Verification items for the finished model (mm, model axes). A direction names the side the tool comes from. Give positions to 0.01 mm unless a question says otherwise; leave off trailing zeros. Loops run counter-clockwise (first coordinate to the right, second up) from the corner with the lowest first, then second, coordinate; pieces in that order, holes last. Notation, with made-up numbers: (18.5, 65.25) -> (46.5, 65.25) arc R9 cw to (46.5, 72.25) -> close; hole circle Ø6 at (4, -8.75). An arc over 180 degrees is marked (long way). Use one line per item in the form item = value. Start each with the question number.
from build123d import *

# Parameters (mm, degrees)
F0_W        = 7.45
F0_H        = 4
F1_DEPTH    = 2
F2_W        = 7.45
F2_H        = 5.9
F3_DEPTH    = 1.75
F6_W        = 7.45
F6_H        = 5
F7_DEPTH    = 2
F8_R        = 0.75
F9_T1_DEPTH = 1.05
F9_S5_W     = 0.75
F9_S5_H     = 0.75
F9_T6_DEPTH = 0.75


# Not quite as in the source:
# - a fillet or chamfer that OpenCascade refuses, or shapes differently, is made with other operations: its cross-section is extruded or revolved along the edge and cut away or added


with BuildPart() as f1:
    # F0 (on Top) → F1 (new body)
    with BuildSketch(Plane.XY):
        with Locations((3.725, 2)):
            Rectangle(F0_W, F0_H)
    extrude(amount=F1_DEPTH)

    # F2 (on face) → F3 (join)
    with BuildSketch(Plane.XY.offset(2)):
        with Locations((3.725, 2.85)):
            Rectangle(F2_W, F2_H)
    extrude(amount=F3_DEPTH)

    # F6 (on line) → F7 (join)
    with BuildSketch(Plane(origin=(0, 2.8829689891, 1.0493148984), x_dir=(-1, 0, 0), z_dir=(0, 0.9396926208, 0.3420201433))):
        with Locations((-3.725, 5.3740090556)):
            Rectangle(F6_W, F6_H)
    extrude(amount=-F7_DEPTH)

    # F8
    f8_edges = [f1.edges().sort_by_distance(p)[0] for p in [
        (7.45, 5.8, 2.875),
        (7.45, 3.85, 3.75),
        (3.725, 5.8, 3.75),
        (3.725, 5.8, 2),
        (0, 5.8, 2.875),
        (0, 3.85, 3.75),
        (0, 4.9, 2),
        (0, 1.04495, 6.099232),
        (3.725, 0.189899, 8.448463),
        (7.45, 1.04495, 6.099232),
        (7.45, -0.749793, 8.106443),
        (0, -0.749793, 8.106443),
    ]]
    fillet(f8_edges, radius=F8_R)

    # F9: fillet of radius 0.75 on 1 edges, made by hand

    # F9_s2 → F9_t1 (cut)
    with BuildSketch(Plane.XZ.offset(-5.05)):
        with BuildLine():
            ThreePointArc((7.45, 2.75), (7.2303300859, 2.2196699141), (6.7, 2))
            Line((6.7, 2), (7.45, 2))
            Line((7.45, 2), (7.45, 2.75))
        make_face()
    extrude(amount=F9_T1_DEPTH, mode=Mode.SUBTRACT)


with BuildPart() as f9_tool4:
    # F9_s5 → F9_t6 (new body)
    with BuildSketch(Plane.YZ.offset(6.7)):
        with Locations((5.425, 2.375)):
            Rectangle(F9_S5_W, F9_S5_H)
    extrude(amount=F9_T6_DEPTH)

    # F9_s7 → F9_t8 (revolve, cut)
    with BuildSketch(Plane(origin=(6.7, 5.05, 2.75), x_dir=(0, -0.7071067812, 0.7071067812), z_dir=(0, 0.7071067812, 0.7071067812))):
        with BuildLine():
            ThreePointArc((0, -0.75), (0.75, 0), (0, 0.75))
            Line((0, 0.75), (0, -0.75))
        make_face()
    revolve(axis=Axis((6.7, 5.05, 2.75), (1, 0, 0)), mode=Mode.SUBTRACT)


with BuildPart() as f1_1:
    add(f1.part)

    # F9_t3: cut F9_tool4
    add(f9_tool4.part, mode=Mode.SUBTRACT)


solid = f1_1.part
Item 1: Gauge pin test, flat ends, axial feed: pin 1 Ø0.8 at (x, z) = (5, 1) entering from +Y; pin 2 Ø1.5 at (x, z) = (2, 3) entering from -Y; pin 3 Ø2 at (x, y) = (6.5, 4) entering from +Z; pin 4 Ø1.2 at (x, y) = (4, 4.5) entering from -Z. Record the tip position at first contact, or that the pin passes through.
Item 2: Tool access check on faces 1 (the flat face through (4, -0.1, 3)), 2 (the flat face through (3.7, 4.5, 2)), 3 (the cylindrical face through (0.21, 1.04, 5.45)), 4 (the flat face through (4, 3, 3.75)), 5 (the cylindrical face through (3.68, 0.07, 8.16)). Record the directions out of +Z, -Z, +X, -X, +Y, -Y that give a thin tool (end or side, any length) a straight path to the whole face; none if there is none.
Item 3: Sectioned sample at A-A, the plane x = 4.25. Enter the section's corners in (y, z), and give its area (3 significant figures).
Item 4: Sectioned sample at B-B, the plane y = 4.5. Enter the section's corners in (x, z).
Item 5: Material ranges on line 1 (Z direction, x = 3.5, y = 2.5); line 2 (Y direction, x = 7.25, z = 1); line 3 (Z direction, x = 4, y = 4.5), recorded low to high.
Item 6: Sectioned sample at C-C, the plane z = 2.5. Enter the section's corners in (x, y), and give its area (3 significant figures).
Outcome:
q1.pin_1 = 4
q1.pin_2 = -0.23
q1.pin_3 = 3.75
q1.pin_4 = 0
q2.face_1 = -Z, +X, -X, -Y
q2.face_2 = -Z, +X, -X, +Y
q2.face_3 = +Z, -X, +Y
q2.face_4 = +Z, +X, -X, +Y
q2.face_5 = +Z, +X, -X
q3.outline = (-1.69, 7.76) -> (-0.1, 3.4) -> (-0.1, 2) -> (0, 2) -> (0, 0) -> (4, 0) -> (4, 2) -> (5.05, 2) arc R0.75 ccw to (5.8, 2.75) -> (5.8, 3) arc R0.75 ccw to (5.05, 3.75) -> (1.9, 3.75) -> (0.45, 7.74) arc R0.75 ccw to (-0.51, 8.19) -> close
q3.area = 27.3 mm^2
q4.outline = (0, 2.75) arc R0.75 ccw to (0.75, 2) -> (6.7, 2) arc R0.75 ccw to (7.45, 2.75) -> (7.45, 3) arc R0.75 ccw to (6.7, 3.75) -> (0.75, 3.75) arc R0.75 ccw to (0, 3) -> close
q5.line_1 = 0 to 3.75
q5.line_2 = 0 to 4
q5.line_3 = 2 to 3.75
q6.outline = (0, -0.1) -> (7.45, -0.1) -> (7.45, 4) -> (7.41, 4) -> (7.41, 5.05) arc R0.71 ccw to (6.7, 5.76) -> (0.75, 5.76) arc R0.71 ccw to (0.04, 5.05) -> (0.04, 4) -> (0, 4) -> close
q6.area = 43.3 mm^2
